Can you work these out from the model? Positions are in its coordinate system, mm. Face numbers are marked on the shaded views. A direction names the side the tool comes from. Give positions to 0.01 mm unless a question says otherwise; leave off trailing zeros. Order: outer loops, then holes, each group sorted by start corner. A loop starts at its lowest first (then second) coordinate and runs counter-clockwise, first axis right, second up. Notation, with made-up numbers: (81, -32.75) - (131, -32.75) arc R23 cw to (131, -2.75) - close; hole circle Ø6 at (40.5, -18.75). An arc over 180 degrees is marked (long way). Answer as a JSON object with one key per item and string values.
```python
from build123d import *

# Parameters (mm, degrees)
SKETCH1_W           = 50
SKETCH1_H           = 58
BOSS_EXTRUDE1_DEPTH = 20
SKETCH2_R           = 2.25
CUT_EXTRUDE1_DEPTH  = 86.813751812
SKETCH3_W           = 44
SKETCH3_H           = 14
CUT_EXTRUDE2_DEPTH  = 53
CHAMFER1_SIZE       = 1


with BuildPart() as part:
    # Sketch1 → Boss-Extrude1 (new body)
    with BuildSketch(Plane.XY):
        with Locations((35, 29)):
            Rectangle(SKETCH1_W, SKETCH1_H)
    extrude(amount=BOSS_EXTRUDE1_DEPTH)

    # Sketch2 → Cut-Extrude1 (cut, through all)
    with BuildSketch(Plane(origin=(0, 58, 0), x_dir=(1, 0, 0), z_dir=(0, 1, 0))):
        with Locations(Location((20, -10, 0), (0, 0, 180))):
            Circle(SKETCH2_R)
        with Locations(Location((50, -10, 0), (0, 0, 180))):
            Circle(SKETCH2_R)
    extrude(amount=-CUT_EXTRUDE1_DEPTH, mode=Mode.SUBTRACT)

    # Sketch3 → Cut-Extrude2 (cut)
    with BuildSketch(Plane.XZ):
        with Locations((35, 10)):
            Rectangle(SKETCH3_W, SKETCH3_H)
    extrude(amount=-CUT_EXTRUDE2_DEPTH, mode=Mode.SUBTRACT)

    # Chamfer1
    chamfer1_edges = [part.edges().sort_by_distance(p)[0] for p in [
        (60, 29, 20),
        (35, 58, 20),
        (60, 29, 0),
        (10, 29, 0),
        (35, 58, 0),
        (60, 58, 10),
        (10, 58, 10),
        (10, 29, 20),
    ]]
    chamfer(chamfer1_edges, length=CHAMFER1_SIZE)


solid = part.part
```
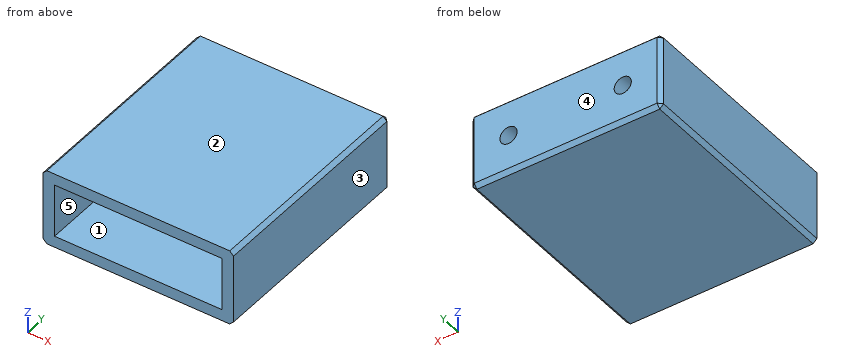
Q1. I'm going to push flat-ended pins straight in: pin 1 Ø3 at (x, z) = (48.5, 7.5) entering from -Y; pin 2 Ø8 at (x, z) = (51, 2) entering from -Y; pin 3 Ø3.5 at (x, z) = (20, 10) entering from +Y. Where does each tip first touch, or does it pass through?
Recorded:
{"pin 1": "stops at y = 53", "pin 2": "stops at y = 0", "pin 3": "passes through"}
Q2. If we section it at D-D, the plane x = 32: Please give me the cut outline in (y, z).
Recorded:
{"outline": "(0, 0) - (57, 0) - (58, 1) - (58, 19) - (57, 20) - (0, 20) - (0, 17) - (53, 17) - (53, 3) - (0, 3) - close"}
Q3. We'd pull the mould along Z, two halves only. Please class the marked faces 1, 2 and 3: released by +Z, released by -Z, zero draft, split by the parting line, or undercut.
Recorded:
{"face 1": "undercut", "face 2": "released by +Z", "face 3": "zero draft"}
Q4. I need wall thicknesses on L1, parallel to Z at x = 20, y = 55.6; L2, parallel to X at y = 9.5, z = 15.75; L3, parallel to Z at x = 28, y = 7.5. Which ranges of each line are inside material? Lowest first, please.
Recorded:
{"L1": "z = 0 to 7.75, 12.25 to 20", "L2": "x = 10 to 13, 57 to 60", "L3": "z = 0 to 3, 17 to 20"}
Q5. If we section it at B-B, the plane y = 42: Please give me the cut outline in (x, z).
Recorded:
{"outline": "(10, 1) - (11, 0) - (59, 0) - (60, 1) - (60, 19) - (59, 20) - (11, 20) - (10, 19) - close; hole (13, 3) - (57, 3) - (57, 17) - (13, 17) - close"}
Q6. Which directions (+Z, -Z, +X, -X, +Y, -Y) give clear straight access to the entire face, cutting with the end or side of a thin tool? Please do the marked faces 4 and 5.
Recorded:
{"face 4": "+Z, -Z, +X, -X, +Y", "face 5": "-Y"}
Q7. If we section it at C-C, the plane x = 20: Please give me the cut outline in (y, z), then the cut area to 4 significant figures.
Recorded:
{"outline": "(0, 0) - (57, 0) - (58, 1) - (58, 7.75) - (53, 7.75) - (53, 3) - (0, 3) - close; (0, 17) - (53, 17) - (53, 12.25) - (58, 12.25) - (58, 19) - (57, 20) - (0, 20) - close", "area": "394.5 mm^2"}
Q8. If we section it at A-A, the plane z = 10: Please give me the cut outline in (x, y).
Recorded:
{"outline": "(10, 0) - (13, 0) - (13, 53) - (17.75, 53) - (17.75, 58) - (11, 58) - (10, 57) - close; (22.25, 53) - (47.75, 53) - (47.75, 58) - (22.25, 58) - close; (52.25, 53) - (57, 53) - (57, 0) - (60, 0) - (60, 57) - (59, 58) - (52.25, 58) - close"}
